Read the model definition and answer for the solid it produces. Units are mm, in the model's axes. Face numbers are marked on the shaded views. A direction names the side the tool comes from. Round coordinates to 2 decimals unless told otherwise and drop trailing zeros. Loops run counter-clockwise (first coordinate to the right, second up) from the corner with the lowest first, then second, coordinate; pieces in that order, holes last. Notation, with made-up numbers: M 65.5,54.25 L 101.5,54.25 A19 ccw 101.5,90.25 Z; hole C -8.5,57.5 d10. An arc over 180 degrees is marked long. Write each question's results on one line, items separated by ' | '.
```python
from build123d import *

# Parameters (mm, degrees)
SKETCH1_W           = 31.5
SKETCH1_H           = 170
SKETCH1_W_2         = 5.08
SKETCH1_H_2         = 150
BOSS_EXTRUDE1_DEPTH = 3.175
FILLET1_R           = 1
FILLET2_R           = 5
BOSS_EXTRUDE2_DEPTH = 70
FILLET3_R           = 15
SKETCH4_W           = 5
SKETCH4_H           = 40
CUT_EXTRUDE5_DEPTH  = 104.989569915


with BuildPart() as part:
    # Sketch1 → Boss-Extrude1 (new body)
    with BuildSketch(Plane.XY):
        Rectangle(SKETCH1_W, SKETCH1_H)
        Rectangle(SKETCH1_W_2, SKETCH1_H_2, mode=Mode.SUBTRACT)
    extrude(amount=BOSS_EXTRUDE1_DEPTH)

    # Fillet1
    fillet1_edges = [part.edges().sort_by_distance(p)[0] for p in [
        (2.54, 75, 1.5875),
        (-2.54, 75, 1.5875),
        (-2.54, -75, 1.5875),
        (2.54, -75, 1.5875),
    ]]
    fillet(fillet1_edges, radius=FILLET1_R)

    # Fillet2
    fillet2_edges = [part.edges().sort_by_distance(p)[0] for p in [
        (15.75, 85, 1.5875),
        (15.75, -85, 1.5875),
        (-15.75, -85, 1.5875),
        (-15.75, 85, 1.5875),
    ]]
    fillet(fillet2_edges, radius=FILLET2_R)

    # Sketch3 → Boss-Extrude2 (add)
    with BuildSketch(Plane(origin=(0, -85, 0), x_dir=(1, 0, 0), z_dir=(0, 1, 0))):
        with BuildLine():
            Line((-56.65, -16.978040594), (-55, -19.483534558))
            ThreePointArc((-55, -19.483534558), (0, -3), (55, -19.483534558))
            Line((55, -19.483534558), (56.65, -16.978040594))
            ThreePointArc((56.65, -16.978040594), (0, 0), (-56.65, -16.978040594))
        make_face()
    extrude(amount=BOSS_EXTRUDE2_DEPTH)

    # Fillet3
    fillet3_edges = [part.edges().sort_by_distance(p)[0] for p in [
        (55.825, -85, 18.230787576),
        (-55.825, -85, 18.230787576),
        (-55.825, -15, 18.230787576),
        (55.825, -15, 18.230787576),
    ]]
    fillet(fillet3_edges, radius=FILLET3_R)

    # Sketch4 → Cut-Extrude5 (cut, symmetric)
    with BuildSketch(Plane.XY):
        with Locations((-44.5945609, -50)):
            Rectangle(SKETCH4_W, SKETCH4_H)
    cut_extrude5 = extrude(amount=CUT_EXTRUDE5_DEPTH, both=True, mode=Mode.SUBTRACT)

    # Mirror1: Cut-Extrude5 across plane
    add(cut_extrude5.mirror(Plane(origin=(0, 0, 0), x_dir=(0, 0, 1), z_dir=(1, 0, 0))), mode=Mode.SUBTRACT)


solid = part.part
```
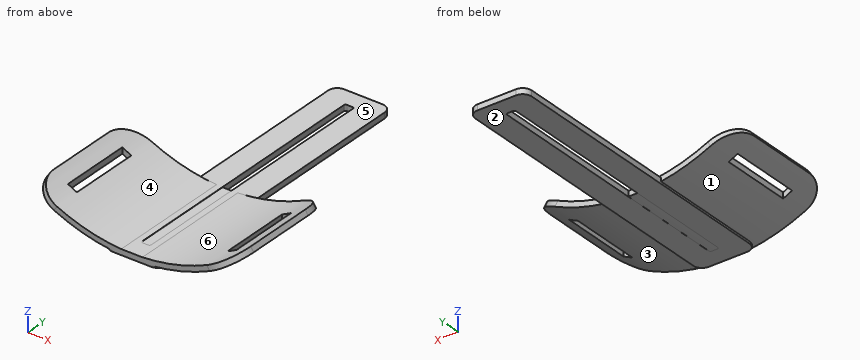
1. Find section D-D, the plane x = -12.5. Give the vertices of the cut face in (y, z) (3 decimals), then the cut area to 3 significant figures.
Completed:
outline: M -85,0.761 L -84.684,0.761 L -84.684,0 L 84.684,0 L 84.684,3.175 L -15,3.175 L -15,3.784 L -85,3.784 Z | area: 581 mm2
2. Find the intervals of material crossed by L1, parallel to Y at x = 21, z = 2.25; L2, parallel to X at y = -64, z = 10.5; L3, parallel to Z at x = 12, y = 74.5 (3 decimals), in increasing order.
Completed:
L1: y = -85 to -15 | L2: x = -42.09 to -38, 38 to 42.09 | L3: z = 0 to 3.175
3. Find section A-A, the plane y = -55. Count the separate pieces of the cut face and the enclosed holes in it, then the cut area to 3 significant figures.
Completed:
separate pieces: 3 | enclosed holes: 0 | area: 334 mm2
4. Which of the six approach directions +Z, -Z, +X, -X, +Y, -Y give full straight-line access (tool end or side, diameter ignored) to the marked faces 5 and 6?
Completed:
face 5: +Z, +Y | face 6: +Z, +Y, -Y
5. Given P1, Ø5, axis at y = -23.5, z = 9, coming from the +X side; P2, Ø3.5, axis at y = -48, z = 12.5, coming from the -X side; P3, Ø2.5, axis at x = 45.5, z = 13, coming from the +Y side; P4, Ø6, axis at x = 41, z = 8, coming from the -Y side, each flat-ended and moving along its own axis, determine where each tip first touches the part or whether it passes through.
Completed:
P1: stops at x = 47.29 | P2: stops at x = -52.27 | P3: stops at y = -15.17 | P4: stops at y = -85
6. Find section B-B, the plane z = 6.75. Give the vertices of the cut face in (x, y), then the cut area to 3 significant figures.
Completed:
outline: M -36.67,-85 L -27.13,-85 L -27.13,-15 L -36.67,-15 Z; M 27.13,-85 L 36.67,-85 L 36.67,-15 L 27.13,-15 Z | area: 1,340 mm2
7. Determine the mould class of the marked faces 1, 2, 3 and 4 for opening direction X: released by +X, released by -X, zero draft, split by the parting line, or undercut.
Completed:
face 1: released by -X | face 2: zero draft | face 3: released by +X | face 4: undercut
8. Find section C-C, the plane y = 31. Give the vertices of the cut face in (x, z) (3 decimals), then the cut area to 3 significant figures.
Completed:
outline: M -15.75,0 L -2.54,0 L -2.54,3.175 L -15.75,3.175 Z; M 2.54,0 L 15.75,0 L 15.75,3.175 L 2.54,3.175 Z | area: 83.9 mm2
